Geometry: see drawing. Coordinates: mm, zero at the bounding-box minimum. Give positions to 0.01 mm unless a question says otherwise; leave off trailing zeros. Loops run counter-clockwise (first coordinate to the right, second up) from the corner with the lowest first, then second, coordinate; pieces in that order, holes last. Notation, with made-up numbers: (17.5, 6.25) - (29.5, 6.25) arc R18 cw to (29.5, 31.25) - close; hole circle Ø9 at (88, 29.5). An arc over 180 degrees is marked (long way). Use CSV: the item, a comma, the result in double quotes. Start each with the question number.
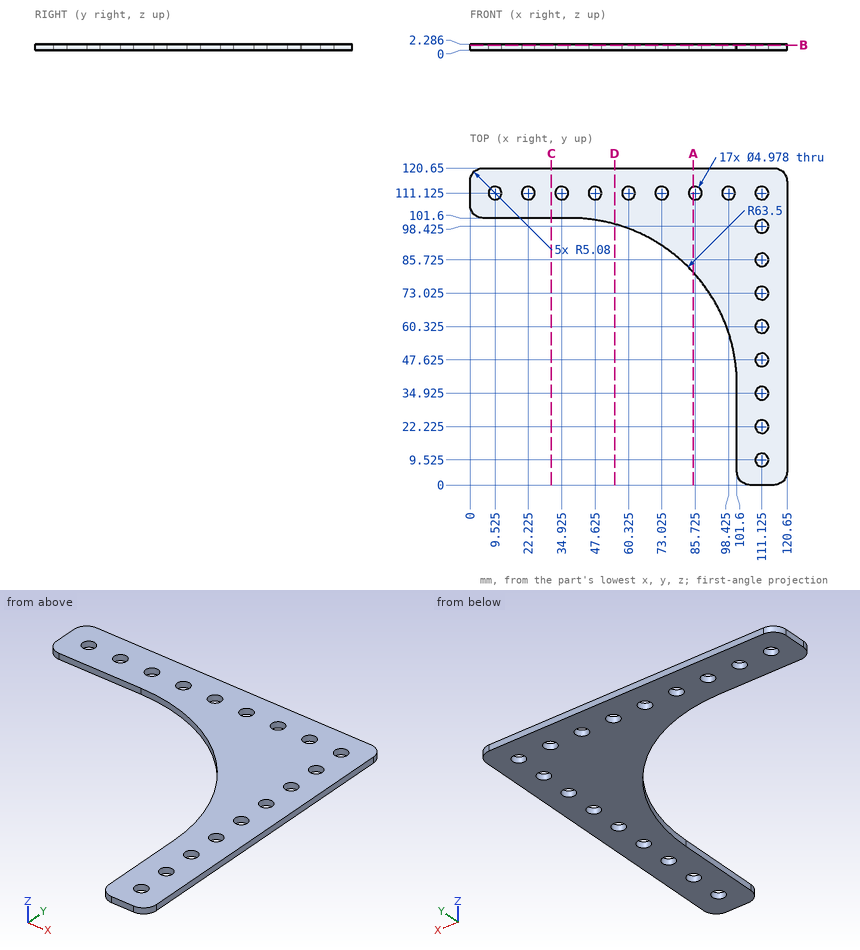
Item 1: Section C-C (x = 31). Output: boundary loops of the cut face in (y, z).
Item 2: Ray query, probe 1 along Y at (x, z) = (21, 0.55); probe 2 along Y at (x, z) = (6.5, 1.8); probe 3 along X at (y, z) = (20.5, 1.3). Return the intervals inside material, ascending.
Item 3: Pin query (flat end, axial travel): pin 1 Ø8 at (x, y) = (60.325, 111.125) entering from -Z. Return the tip coordinate at first contact, or that it passes through.
Item 4: Section B-B (z = 1.85). Give the number of separate pieces and of enclosed holes in the cut face, plus the area to 3 significant figures.
Item 5: Section D-D (x = 55). Output: boundary loops of the cut face in (y, z).
Item 6: Section A-A (x = 85). Output: boundary loops of the cut face in (y, z).
Outcome:
1,outline,"(101.6, 0) - (120.65, 0) - (120.65, 2.29) - (101.6, 2.29) - close"
2,probe 1,"y = 101.6 to 108.96, 113.29 to 120.65"
2,probe 2,"y = 101.6 to 120.65"
2,probe 3,"x = 101.6 to 109.33, 112.92 to 120.65"
3,pin 1,"stops at z = 0"
4,separate pieces,"1"
4,enclosed holes,"17"
4,area,"4,740 mm2"
5,outline,"(99.31, 0) - (120.65, 0) - (120.65, 2.29) - (99.31, 2.29) - close"
6,outline,"(80.91, 0) - (108.74, 0) - (108.74, 2.29) - (80.91, 2.29) - close; (113.51, 0) - (120.65, 0) - (120.65, 2.29) - (113.51, 2.29) - close"
